```python
from build123d import *

# Parameters (mm, degrees)
RESSALTO_EXTRUS_O1_DEPTH = 12.7
ESBO_O2_R                = 2.5
CORTE_EXTRUS_O1_DEPTH    = 142.372875758
ESBO_O3_R                = 2.5
CORTE_EXTRUS_O2_DEPTH    = 143.311383944
FILETE1_R                = 5
FILETE2_R                = 5


with BuildPart() as part:
    # Esboço1 → Ressalto-extrusão1 (new body)
    with BuildSketch(Plane.XY):
        with BuildLine():
            Line((0, 0), (37.639320225, 0))
            ThreePointArc((37.639320225, 0), (39.93684943, 0.267510105), (42.11145618, 1.05572809))
            Line((42.11145618, 1.05572809), (117.88854382, 38.94427191))
            ThreePointArc((117.88854382, 38.94427191), (120.06315057, 39.732489895), (122.360679775, 40))
            Line((122.360679775, 40), (135, 40))
            Line((135, 40), (135, 43.2))
            Line((135, 43.2), (122.360679775, 43.2))
            ThreePointArc((122.360679775, 43.2), (119.327941224, 42.846886661), (116.457460314, 41.806438921))
            Line((116.457460314, 41.806438921), (40.680372674, 3.917895101))
            ThreePointArc((40.680372674, 3.917895101), (39.201640085, 3.381906872), (37.639320225, 3.2))
            Line((37.639320225, 3.2), (0, 3.2))
            Line((0, 3.2), (0, 0))
        make_face()
    extrude(amount=RESSALTO_EXTRUS_O1_DEPTH)

    # Esboço2 → Corte-extrusão1 (cut, through all)
    with BuildSketch(Plane(origin=(0, 3.2, 0), x_dir=(1, 0, 0), z_dir=(0, 1, 0))):
        with Locations(Location((6, -6.35, 0), (0, 0, 270))):
            Circle(ESBO_O2_R)
        with Locations(Location((31, -6.35, 0), (0, 0, 270))):
            Circle(ESBO_O2_R)
    extrude(amount=-CORTE_EXTRUS_O1_DEPTH, mode=Mode.SUBTRACT)

    # Esboço3 → Corte-extrusão2 (cut, through all)
    with BuildSketch(Plane(origin=(0, 43.2, 0), x_dir=(1, 0, 0), z_dir=(0, 1, 0))):
        with Locations(Location((128.680339887, -6.35, 0), (0, 0, 270))):
            Circle(ESBO_O3_R)
    extrude(amount=-CORTE_EXTRUS_O2_DEPTH, mode=Mode.SUBTRACT)

    # Filete1
    filete1_edges = [part.edges().sort_by_distance(p)[0] for p in [
        (135, 41.6, 12.7),
    ]]
    fillet(filete1_edges, radius=FILETE1_R)

    # Filete2
    filete2_edges = [part.edges().sort_by_distance(p)[0] for p in [
        (135, 41.6, 0),
    ]]
    fillet(filete2_edges, radius=FILETE2_R)


solid = part.part
```
The listing builds one solid part. Answer for the finished solid, in the listing's coordinates (mm). A direction names the side the tool comes from. Round coordinates to 2 decimals unless told otherwise and drop trailing zeros. Loops run counter-clockwise (first coordinate to the right, second up) from the corner with the lowest first, then second, coordinate; pieces in that order, holes last. Notation, with made-up numbers: (13.25, 17.25) - (22.25, 17.25) arc R24 cw to (22.25, 49.25) - close; hole circle Ø11 at (22, -13). An arc over 180 degrees is marked (long way). Return JSON: item names as keys, results as strings. Group by question number.
1. Each of these flat-tipped pins is pushed along its axis until it touches: P1, Ø3, axis at x = 18.5, z = 8, coming from the -Y side; P2, Ø4, axis at x = 128.68, z = 6.35, coming from the +Y side; P3, Ø1, axis at y = 12, z = 9, coming from the -X side; P4, Ø6, axis at y = 17.5, z = 6.5, coming from the +X side. Where does it stop, or does it pass through?
2. Which of the six approach directions +Z, -Z, +X, -X, +Y, -Y give full straight-line access (tool end or side, diameter ignored) to faces 4 (the flat face through (19, 3.2, 6)), 5 (the cylindrical face through (6.11, 1.622, 3.852))?
3. The part is cut by section D-D on x = 104. Determine the outline of the cut face in (y, z).
4. The mould has two halves that part along Z. Classify faces 1 (the flat face through (65, 15, 0)), 2 (the cylindrical face through (126.24, 41.62, 5.81)), 3 (the flat face through (126, 40, 6)): pulls with the +Z half, pulls with the -Z half, needs draft (parallel to the pull), parting line crosses it, or undercut.
5. The part is cut by section A-A on z = 6.35. Determine the outline of the cut face in (x, y), then the cut area to 3 significant figures.
6. The part is cut by section C-C on y = 23.5. Determine the outline of the cut face in (x, z).
7. The part is cut by section B-B on x = 31. Determine the outline of the cut face in (y, z).
8. Consider probe 1 along X at (y, z) = (1.7, 6.35); probe 2 along Y at (x, z) = (12, 3); probe 3 along Y at (x, z) = (127, 2.5). Determine where each line is inside the solid, lowest interval first.
Resolved:
{
 "1": {"P1": "stops at y = 0", "P2": "passes through", "P3": "stops at x = 55.84", "P4": "stops at x = 81"},
 "2": {"face 4": "+Z, -Z, -X, +Y", "face 5": "+Y, -Y"},
 "3": {"outline": "(32, 0) - (35.58, 0) - (35.58, 12.7) - (32, 12.7) - close"},
 "4": {"face 1": "pulls with the -Z half", "face 2": "undercut", "face 3": "needs draft"},
 "5": {"outline": "(0, 0) - (3.5, 0) - (3.5, 3.2) - (0, 3.2) - close; (8.5, 0) - (28.5, 0) - (28.5, 3.2) - (8.5, 3.2) - close; (33.5, 0) - (37.64, 0) arc R10 ccw to (42.11, 1.06) - (117.89, 38.94) arc R10 cw to (122.36, 40) - (126.18, 40) - (126.18, 43.2) - (122.36, 43.2) arc R13.2 ccw to (116.46, 41.81) - (40.68, 3.92) arc R6.8 cw to (37.64, 3.2) - (33.5, 3.2) - close; (131.18, 40) - (135, 40) - (135, 43.2) - (131.18, 43.2) - close", "area": "414 mm²"},
 "6": {"outline": "(79.84, 0) - (87, 0) - (87, 12.7) - (79.84, 12.7) - close"},
 "7": {"outline": "(0, 0) - (3.2, 0) - (3.2, 3.85) - (0, 3.85) - close; (0, 8.85) - (3.2, 8.85) - (3.2, 12.7) - (0, 12.7) - close"},
 "8": {"probe 1": "x = 0 to 3.5, 8.5 to 28.5, 33.5 to 43.4", "probe 2": "y = 0 to 3.2", "probe 3": "y = 40 to 43.2"}
}
